```python
from build123d import *

# Parameters (mm, degrees)
EXTRUDE_THIN1_DEPTH = 158.75
FILLET1_R           = 1.9812


with BuildPart() as part:
    # Sketch1 → Extrude-Thin1 (new body)
    with BuildSketch(Plane.XY):
        with BuildLine():
            Line((0, 0), (-9.525, 0))
            Line((-9.525, 0), (-9.525, 8.73125))
            ThreePointArc((-9.525, 8.73125), (-5.250982158, 11.13965279), (-3.96875, 15.875))
            Line((-3.96875, 15.875), (0, 15.875))
            Line((0, 15.875), (0, 13.8938))
            Line((0, 13.8938), (-2.011138875, 13.8938))
            ThreePointArc((-2.011138875, 13.8938), (-3.827545416, 9.747705801), (-7.5438, 7.163352557))
            Line((-7.5438, 7.163352557), (-7.5438, 1.9812))
            Line((-7.5438, 1.9812), (0, 1.9812))
            Line((0, 1.9812), (0, 0))
        make_face()
    extrude(amount=-EXTRUDE_THIN1_DEPTH)

    # Fillet1
    fillet1_edges = [part.edges().sort_by_distance(p)[0] for p in [
        (-9.525, 0, -79.375),
        (-9.525, 8.73125, -79.375),
        (-3.96875, 15.875, -79.375),
    ]]
    fillet(fillet1_edges, radius=FILLET1_R)


solid = part.part
```
Geometry check sheet. Reference: the model listing, model coordinates, mm. A direction names the side the tool comes from. Round coordinates to 2 decimals unless told otherwise and drop trailing zeros. Loops run counter-clockwise (first coordinate to the right, second up) from the corner with the lowest first, then second, coordinate; pieces in that order, holes last. Notation, with made-up numbers: (-24, 87) - (-4, 87) arc R8 ccw to (-4, 91) - close; hole circle Ø2 at (-18, 25.25). An arc over 180 degrees is marked (long way). Use a Markdown table: item, result.
Q1. Access from +Z, -Z, +X, -X, +Y, -Y to the whole of each face (thin tool, end or side, straight path). Record for faces 1 (the flat face through (-7.544, 5, -78)), 2 (the flat face through (-6.2, 8, 0)).
Solutions:
| item | result |
|---|---|
| face 1 | +Z, -Z, +X |
| face 2 | +Z, +X, -X, +Y, -Y |
Q2. Draft check along Y on faces 3 (the flat face through (-4, 0, -78)), 4 (the flat face through (-4, 1.981, -78)), 5 (the flat face through (-6.2, 8, -158.75)). Enter one of: released by +Y, released by -Y, zero draft, split by the parting line, or undercut.
Solutions:
| item | result |
|---|---|
| face 3 | released by -Y |
| face 4 | undercut |
| face 5 | zero draft |
Q3. Material ranges on line 1 (Y direction, x = -1.75, z = -46) (3 decimals); line 2 (Y direction, x = -3.25, z = -150); line 3 (X direction, y = 14.25, z = -38), recorded low to high.
Solutions:
| item | result |
|---|---|
| line 1 | y = 0 to 1.981, 13.894 to 15.875 |
| line 2 | y = 0 to 1.98, 10.54 to 15.44 |
| line 3 | x = -3.96 to 0 |
Q4. Go/stop test with flat-tipped pins: P1, Ø5, axis at y = 9, z = -68.5, coming from the +X side; P2, Ø5.5, axis at y = 5, z = -78, coming from the +X side; P3, Ø6, axis at y = 11, z = -40, coming from the -X side. Record where each tip stops, or that it passes through.
Solutions:
| item | result |
|---|---|
| P1 | stops at x = -2.72 |
| P2 | stops at x = -6.23 |
| P3 | stops at x = -9.34 |
Q5. Cross-section at A-A on z = -20.5. Record the cut outline in (x, y) (3 decimals), plus the area to 3 significant figures.
Solutions:
| item | result |
|---|---|
| outline | (-9.525, 1.981) arc R1.981 ccw to (-7.544, 0) - (0, 0) - (0, 1.981) - (-7.544, 1.981) - (-7.544, 7.163) arc R8.331 ccw to (-2.011, 13.894) - (0, 13.894) - (0, 15.875) - (-2.011, 15.875) arc R1.981 ccw to (-3.974, 14.166) arc R6.35 cw to (-8.191, 9.036) arc R1.981 ccw to (-9.525, 7.163) - close |
| area | 53.5 mm2 |
